The figure shows three views and two pictorial views of one solid part (mm, origin at its lowest corner). Answer the questions. A direction names the side the tool comes from. Coordinates: 2 decimals unless noted, no trailing zeros. Order: outer loops, then holes, each group sorted by start corner. A loop starts at its lowest first (then second) coordinate and runs counter-clockwise, first axis right, second up. Notation, with made-up numbers: (57.25, 4.5) - (66.25, 4.5) arc R21 cw to (66.25, 30.5) - close; hole circle Ø6 at (-38, 68). An arc over 180 degrees is marked (long way). Use one line per item in the form item = value.
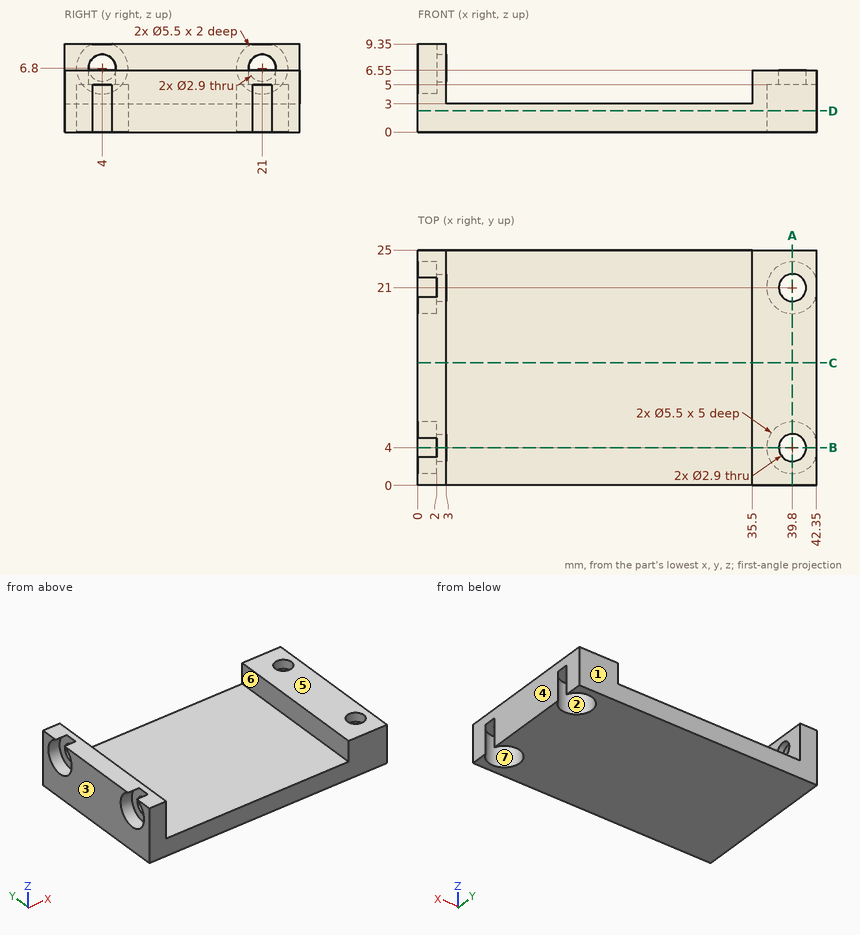
(1) Section B-B, the plane y = 4 is taken. Write down the section's boundary in (x, z).
Answer list:
outline = (0, 0) - (37.05, 0) - (37.05, 5) - (38.35, 5) - (38.35, 6.55) - (35.5, 6.55) - (35.5, 3) - (3, 3) - (3, 5.35) - (2, 5.35) - (2, 4.05) - (0, 4.05) - close; (2, 8.25) - (3, 8.25) - (3, 9.35) - (2, 9.35) - close; (41.25, 5) - (42.35, 5) - (42.35, 6.55) - (41.25, 6.55) - close
(2) Given pin 1 Ø6 at (x, y) = (21, 5.5) entering from +Z; pin 2 Ø2.5 at (x, y) = (39.8, 21) entering from +Z; pin 3 Ø1.6 at (x, y) = (38.5, 3) entering from -Z; pin 4 Ø3.5 at (x, y) = (38.5, 11.5) entering from +Z, each flat-ended and moving along its own axis, determine where each tip first touches the part or whether it passes through.
Answer list:
pin_1 = 3
pin_2 = through
pin_3 = 5
pin_4 = 6.55
(3) Straight lines are drawn through the part: L1, parallel to Y at x = 39.8, z = 2.7; L2, parallel to Y at x = 39.8, z = 5.7; L3, parallel to X at y = 10, z = 5.75. For each, find the intervals that lie inside material, in ascending order.
Answer list:
L1 = 0 to 1.25, 6.75 to 18.25, 23.75 to 25
L2 = 0 to 2.55, 5.45 to 19.55, 22.45 to 25
L3 = 0 to 3, 35.5 to 42.35
(4) The mould has two halves that part along X. Classify the marked faces 1, 2, 3 and 4: +X half, -X half, draft (parallel to the pull), parting line (faces both ways), or undercut.
Answer list:
face_1 = draft
face_2 = undercut
face_3 = -X half
face_4 = +X half
(5) Which of the six approach directions +Z, -Z, +X, -X, +Y, -Y give full straight-line access (tool end or side, diameter ignored) to the marked faces 5, 6 and 7?
Answer list:
face_5 = +Z, +X, +Y, -Y
face_6 = +Z, +Y, -Y
face_7 = -Z
(6) Section C-C, the plane y = 13 is taken. Write down the section's boundary in (x, z), then the cut area to 3 significant figures.
Answer list:
outline = (0, 0) - (42.35, 0) - (42.35, 6.55) - (35.5, 6.55) - (35.5, 3) - (3, 3) - (3, 9.35) - (0, 9.35) - close
area = 170 mm2
(7) Section D-D, the plane z = 2.25 is taken. Write down the section's boundary in (x, y), then the cut area to 3 significant figures.
Answer list:
outline = (0, 0) - (42.35, 0) - (42.35, 2.97) arc R2.75 cw (long way) to (42.35, 5.03) - (42.35, 19.97) arc R2.75 cw (long way) to (42.35, 22.03) - (42.35, 25) - (0, 25) - close
area = 1,010 mm2
(8) Section A-A, the plane x = 39.8 is taken. Write down the section's boundary in (y, z).
Answer list:
outline = (0, 0) - (1.25, 0) - (1.25, 5) - (2.55, 5) - (2.55, 6.55) - (0, 6.55) - close; (5.45, 5) - (6.75, 5) - (6.75, 0) - (18.25, 0) - (18.25, 5) - (19.55, 5) - (19.55, 6.55) - (5.45, 6.55) - close; (22.45, 5) - (23.75, 5) - (23.75, 0) - (25, 0) - (25, 6.55) - (22.45, 6.55) - close
